Verification items for the finished model (mm, model axes). A direction names the side the tool comes from. Give positions to 0.01 mm unless a question says otherwise; leave off trailing zeros. Order: outer loops, then holes, each group sorted by start corner. A loop starts at its lowest first (then second) coordinate and runs counter-clockwise, first axis right, second up.
from build123d import *

# Parameters (mm, degrees)
SKETCH1_W           = 40
SKETCH1_H           = 80
BOSS_EXTRUDE1_DEPTH = 2
BOSS_EXTRUDE2_DEPTH = 80
SKETCH3_R           = 1.3
SKETCH3_W           = 10
SKETCH3_H           = 5
CUT_EXTRUDE1_DEPTH  = 2


with BuildPart() as part:
    # Sketch1 → Boss-Extrude1 (new body)
    with BuildSketch(Plane(origin=(0, 0, 0), x_dir=(1, 0, 0), z_dir=(0, 1, 0))):
        with Locations((20, 40)):
            Rectangle(SKETCH1_W, SKETCH1_H)
    extrude(amount=BOSS_EXTRUDE1_DEPTH)

    # Sketch2 → Boss-Extrude2 (add)
    with BuildSketch(Plane.XY):
        Polygon((0, 2), (-5, 2), (-5, -3), (-3, -3), (-3, 0), (0, 0), align=None)
        Polygon((43, 0), (40, 0), (40, 2), (45, 2), (45, -3), (43, -3), align=None)
    extrude(amount=-BOSS_EXTRUDE2_DEPTH)

    # Sketch3 → Cut-Extrude1 (cut)
    with BuildSketch(Plane(origin=(0, 2, 0), x_dir=(1, 0, 0), z_dir=(0, 1, 0))):
        with Locations(Location((11, 45.5, 0), (0, 0, 270))):
            Circle(SKETCH3_R)
        with Locations(Location((11, 34.5, 0), (0, 0, 270))):
            Circle(SKETCH3_R)
        with Locations(Location((29, 45.5, 0), (0, 0, 90))):
            Circle(SKETCH3_R)
        with Locations(Location((29, 34.5, 0), (0, 0, 90))):
            Circle(SKETCH3_R)
        with Locations((20, 57)):
            Rectangle(SKETCH3_W, SKETCH3_H)
    extrude(amount=-CUT_EXTRUDE1_DEPTH, mode=Mode.SUBTRACT)


solid = part.part
(1) Section check A-A, the plane x = 22. Enter the section's corners in (y, z).
Solved:
outline: (0, -80) - (2, -80) - (2, -59.5) - (0, -59.5) - close; (0, -54.5) - (2, -54.5) - (2, 0) - (0, 0) - close
(2) Release check for a two-part mould opening along Z. For faces 1 (the flat face through (20, 1, -54.5)), 2 (the flat face through (20, 2, -39)), 3 (the flat face through (20, 1, -80)), 4 (the cylindrical face through (28.94, 1.01, -44.2)) record: pulls with the +Z half, pulls with the -Z half, needs draft (parallel to the pull), parting line crosses it, or undercut.
Solved:
face 1: undercut
face 2: needs draft
face 3: pulls with the -Z half
face 4: undercut
(3) Set-up check for faces 5 (the flat face through (44, -3, -39)), 6 (the flat face through (43, -2, -39)), 7 (the flat face through (25, 1, -57)): record each of +Z, -Z, +X, -X, +Y, -Y from which the full face is reachable in a straight line by a thin tool's end or side.
Solved:
face 5: +Z, -Z, +X, -X, -Y
face 6: +Z, -Z, -Y
face 7: +Y, -Y
(4) Scan lines: line 1 (Z direction, x = 29, y = 1.65); line 2 (X direction, y = 0.45, z = -34.5); line 3 (X direction, y = -0.4, z = -22). Record each from-to range of solid material in increasing order.
Solved:
line 1: z = -80 to -46.8, -44.2 to -35.8, -33.2 to 0
line 2: x = -5 to 9.7, 12.3 to 27.7, 30.3 to 45
line 3: x = -5 to -3, 43 to 45
(5) Section check C-C, the plane z = -45.5. Enter the section's corners in (x, y), then the cut area to 3 significant figures.
Solved:
outline: (-5, -3) - (-3, -3) - (-3, 0) - (9.7, 0) - (9.7, 2) - (-5, 2) - close; (12.3, 0) - (27.7, 0) - (27.7, 2) - (12.3, 2) - close; (30.3, 0) - (43, 0) - (43, -3) - (45, -3) - (45, 2) - (30.3, 2) - close
area: 102 mm2
(6) Go/stop test with flat-tipped pins: pin 1 (1 mm diameter, centred on x = 35.5, y = -2, fed in from -Z); pin 2 (14 mm diameter, centred on x = 16, z = -32, fed in from -Y). Record where each tip stops, or that it passes through.
Solved:
pin 1: passes through
pin 2: stops at y = 0
(7) Section check B-B, the plane y = 1.2. Enter the section's corners in (x, z), then the cut area to 3 significant figures.
Solved:
outline: (-5, -80) - (45, -80) - (45, 0) - (-5, 0) - close; hole circle Ø2.6 at (11, -45.5); hole circle Ø2.6 at (11, -34.5); hole (15, -59.5) - (25, -59.5) - (25, -54.5) - (15, -54.5) - close; hole circle Ø2.6 at (29, -45.5); hole circle Ø2.6 at (29, -34.5)
area: 3,930 mm2
(8) Section check D-D, the plane x = 29. Enter the section's corners in (y, z).
Solved:
outline: (0, -80) - (2, -80) - (2, -46.8) - (0, -46.8) - close; (0, -44.2) - (2, -44.2) - (2, -35.8) - (0, -35.8) - close; (0, -33.2) - (2, -33.2) - (2, 0) - (0, 0) - close
